The drawing under review shows one solid part. Ordinate dimensions are in mm from its lowest x, y, z. Coordinates: 2 decimals unless noted, no trailing zeros. Loops run counter-clockwise (first coordinate to the right, second up) from the corner with the lowest first, then second, coordinate; pieces in that order, holes last. Notation, with made-up numbers: M 58.5,1 L 77.5,1 A9 ccw 77.5,6 Z; hole C -16.75,10.5 d4. An arc over 180 degrees is marked long. Answer as a JSON object with one key per item and string values. Group by question number.
1. Consider section B-B (y = 1.85). Count the separate pieces of the cut face and the enclosed holes in it, then the cut area to 3 significant figures.
2. Consider section D-D (z = 52). State the section outline as (x, y) points (3 decimals), then the cut area to 3 significant figures.
3. To check wall thickness, follow probe 1 along Z at (x, y) = (4.75, 1.9); probe 2 along X at (y, z) = (0.7, 87.25). State the ranges of each line that lie inside material, in increasing order.
4. Consider section C-C (x = 4.75). State the section outline as (y, z) points, then the cut area to 3 significant figures.
5. Consider section A-A (z = 4.75). State the section outline as (x, y) points.
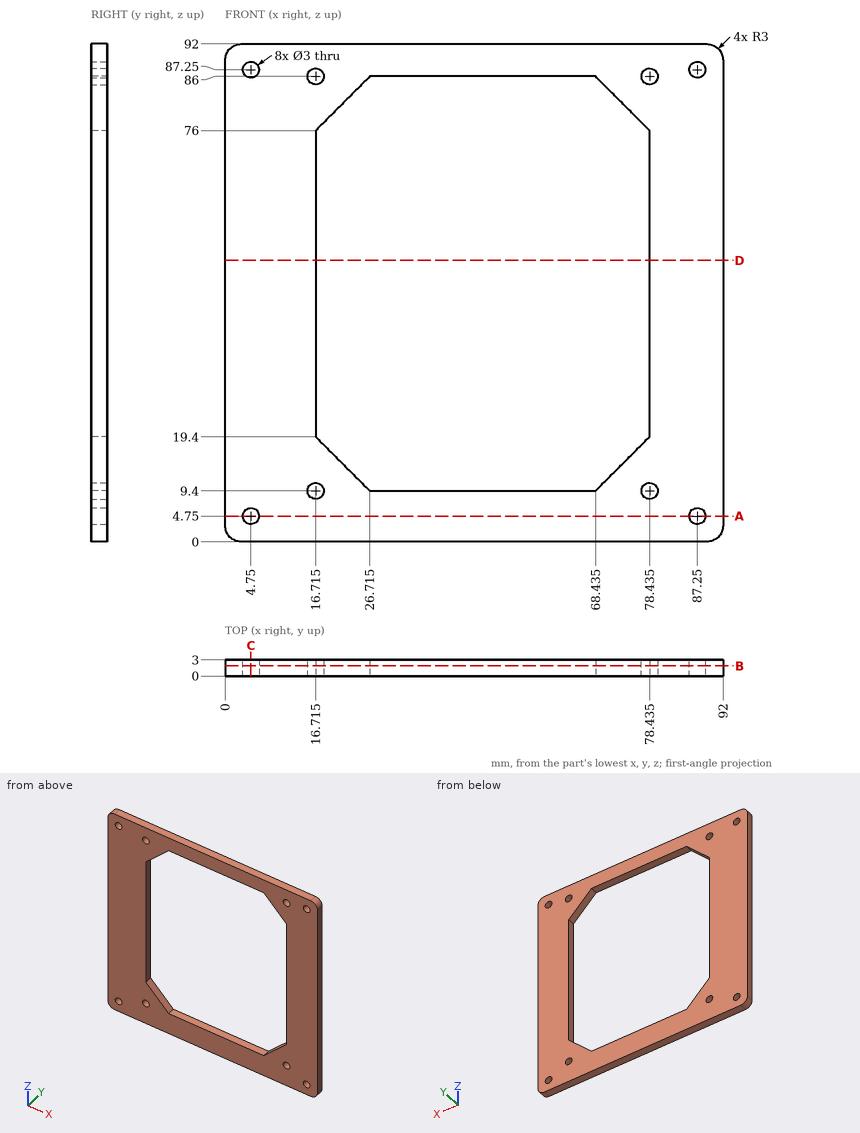
Findings below:
{
 "1": {"separate pieces": "1", "enclosed holes": "9", "area": "3,870 mm^2"},
 "2": {"outline": "M 0,0 L 16.715,0 L 16.715,3 L 0,3 Z; M 78.435,0 L 92,0 L 92,3 L 78.435,3 Z", "area": "90.8 mm^2"},
 "3": {"probe 1": "z = 0 to 3.25, 6.25 to 85.75, 88.75 to 92", "probe 2": "x = 0 to 3.25, 6.25 to 15.89, 17.54 to 77.61, 79.26 to 85.75, 88.75 to 92"},
 "4": {"outline": "M 0,0 L 3,0 L 3,3.25 L 0,3.25 Z; M 0,6.25 L 3,6.25 L 3,85.75 L 0,85.75 Z; M 0,88.75 L 3,88.75 L 3,92 L 0,92 Z", "area": "258 mm^2"},
 "5": {"outline": "M 0,0 L 3.25,0 L 3.25,3 L 0,3 Z; M 6.25,0 L 85.75,0 L 85.75,3 L 6.25,3 Z; M 88.75,0 L 92,0 L 92,3 L 88.75,3 Z"}
}
